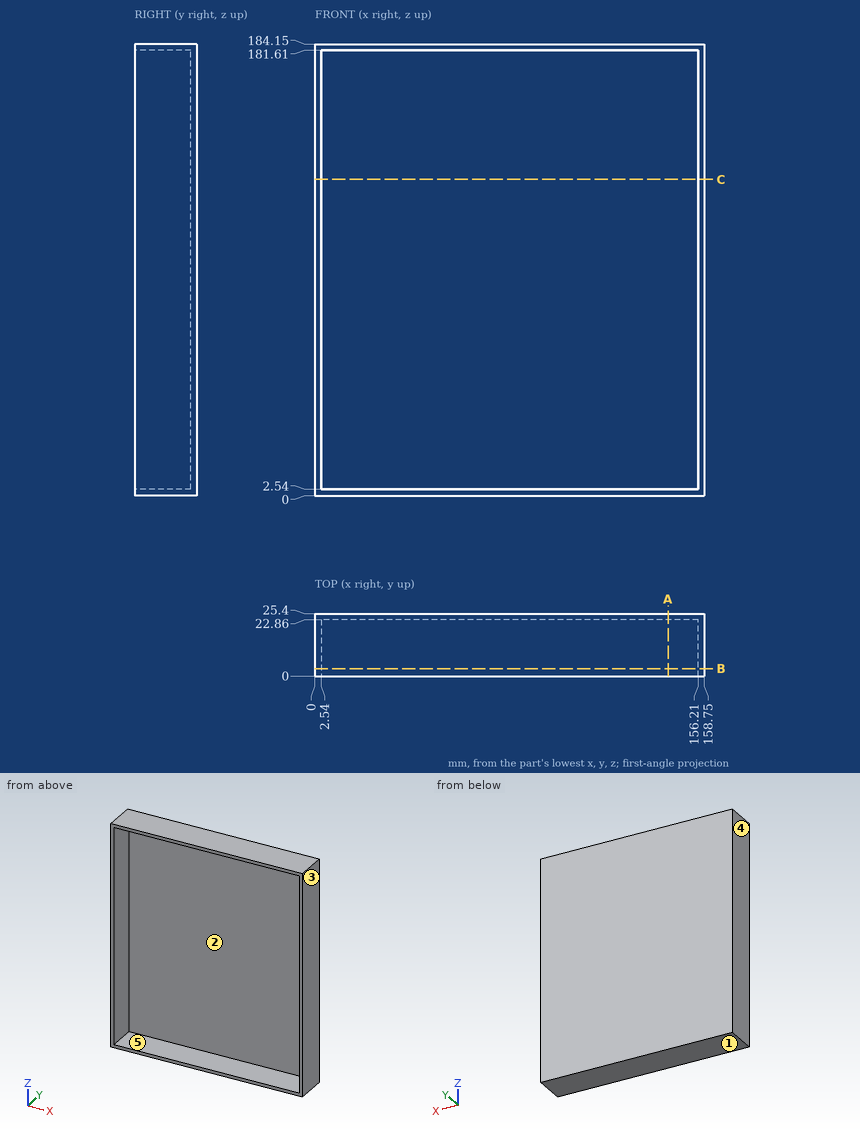
Verification items for this drawing (mm, ordinates from the low corner). A direction names the side the tool comes from. Give positions to 0.01 mm unless a question says otherwise; leave off trailing zeros. Write each loop counter-clockwise with the first axis right and the second up, starting at its lowest first coordinate (ties: lowest second). Pieces come first, ordered by that corner, then holes. Notation, with made-up numbers: (19.5, 69) -> (70.5, 69) arc R27 cw to (70.5, 98) -> close; hole circle Ø5 at (-1, 32.25). An arc over 180 degrees is marked (long way). Use CSV: the item, a comma, the result in double quotes. Start each with the question number.
Q1. Depth check by flat-ended pin: P1, Ø12, axis at x = 78, z = 20, coming from the -Y side. Enter the tip coordinate at first touch or a pass-through.
Q2. Cross-section at C-C on z = 129. Enter the section's corners in (x, y).
Q3. Cross-section at B-B on y = 3. Enter the section's corners in (x, z).
Q4. Scan lines: line 1 along Z through (x, y) = (19.5, 17); line 2 along X through (y, z) = (20.75, 153); line 3 along Y through (x, z) = (108, 163). Record each from-to range of solid material in increasing order.
Q5. Release check for a two-part mould opening along Z. For the marked faces 1, 2 and 3 record: +Z half, -Z half, draft (parallel to the pull), parting line (faces both ways), or undercut.
Q6. Tool access check on the marked faces 4 and 5. Record the directions out of +Z, -Z, +X, -X, +Y, -Y that give a thin tool (end or side, any length) a straight path to the whole face; none if there is none.
Q7. Cross-section at A-A on x = 144. Enter the section's corners in (y, z).
Working result:
1,P1,"stops at y = 22.86"
2,outline,"(0, 0) -> (2.54, 0) -> (2.54, 22.86) -> (156.21, 22.86) -> (156.21, 0) -> (158.75, 0) -> (158.75, 25.4) -> (0, 25.4) -> close"
3,outline,"(0, 0) -> (158.75, 0) -> (158.75, 184.15) -> (0, 184.15) -> close; hole (2.54, 2.54) -> (156.21, 2.54) -> (156.21, 181.61) -> (2.54, 181.61) -> close"
4,line 1,"z = 0 to 2.54, 181.61 to 184.15"
4,line 2,"x = 0 to 2.54, 156.21 to 158.75"
4,line 3,"y = 22.86 to 25.4"
5,face 1,"-Z half"
5,face 2,"undercut"
5,face 3,"draft"
6,face 4,"+Z, -Z, -X, +Y, -Y"
6,face 5,"-Y"
7,outline,"(0, 0) -> (25.4, 0) -> (25.4, 184.15) -> (0, 184.15) -> (0, 181.61) -> (22.86, 181.61) -> (22.86, 2.54) -> (0, 2.54) -> close"
